The drawing under review shows one solid part. Ordinate dimensions are in mm from its lowest x, y, z. A direction names the side the tool comes from. Round coordinates to 2 decimals unless told otherwise and drop trailing zeros. Write each loop counter-clockwise with the first axis right and the second up, starting at its lowest first coordinate (ties: lowest second). Pieces come first, ordered by that corner, then holes. Notation, with made-up numbers: M 42.5,-24.5 L 79.5,-24.5 A28 cw 79.5,-4.5 Z; hole C 8,87 d10. An arc over 180 degrees is marked long. Write item = value, one per line. Start each with the question number.
Item 1: To check wall thickness, follow line 1 along Z through (x, y) = (5, 4); line 2 along Y through (x, z) = (3.5, 6); line 3 along X through (y, z) = (6, 6.25). State the ranges of each line that lie inside material, in increasing order.
Item 2: Take a section at D-D, the plane x = 1.5. Give the boundary of the cut face in (y, z), plus the area to 3 significant figures.
Item 3: Tool access review of the marked faces 1 and 2: name each direction out of +Z, -Z, +X, -X, +Y, -Y from which nothing blocks a thin tool from reaching the whole face with its end or side.
Item 4: For pin 1 Ø2 at (y, z) = (1, 1.5) entering from -X; pin 2 Ø4 at (x, y) = (4, 7) entering from +Z; pin 3 Ø1.5 at (x, y) = (4.5, 7) entering from -Z, all flat-tipped, find the tip position at first contact; note any pin that passes through.
Item 5: Take a section at C-C, the plane z = 5. Give the boundary of the cut face in (x, y).
Item 6: Take a section at B-B, the plane y = 7.75. Give the boundary of the cut face in (x, z), plus the area to 3 significant figures.
Item 7: Take a section at A-A, the plane x = 5. Give the boundary of the cut face in (y, z), plus the area to 3 significant figures.
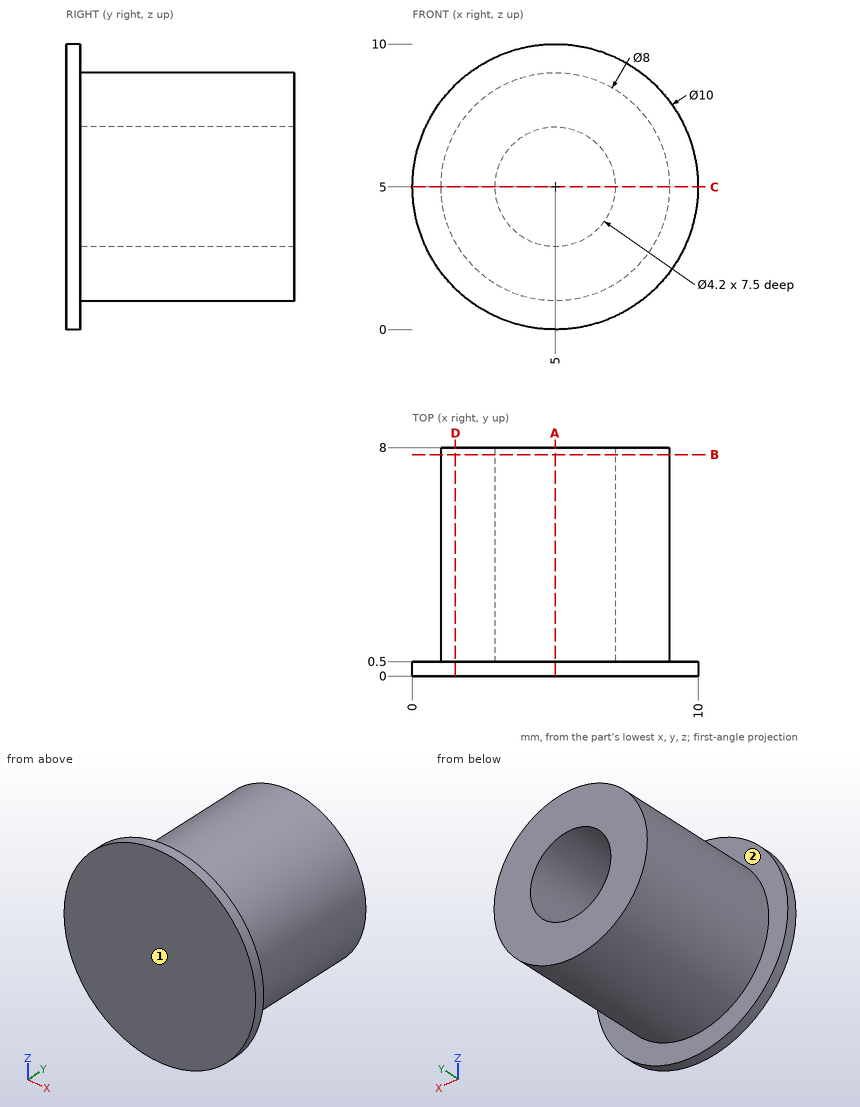
Response values:
q1.line_1 = 1 to 2.9, 7.1 to 9
q1.line_2 = 0 to 0.5
q1.line_3 = 1.2 to 3.31, 6.69 to 8.8
q2.outline = M 0,1.43 L 0.5,1.43 L 0.5,3.06 L 8,3.06 L 8,6.94 L 0.5,6.94 L 0.5,8.57 L 0,8.57 Z
q2.area = 32.6 mm2
q3.face_1 = +Z, -Z, +X, -X, -Y
q3.face_2 = +Y
q4.pin_1 = 0.75
q4.pin_2 = 9
q4.pin_3 = 1
q5.outline = M 0,0 L 10,0 L 10,0.5 L 9,0.5 L 9,8 L 7.1,8 L 7.1,0.5 L 2.9,0.5 L 2.9,8 L 1,8 L 1,0.5 L 0,0.5 Z
q6.outline = C 5,5 d8; hole C 5,5 d4.2
q6.area = 36.4 mm2
q7.outline = M 0,0 L 0.5,0 L 0.5,1 L 8,1 L 8,2.9 L 0.5,2.9 L 0.5,7.1 L 8,7.1 L 8,9 L 0.5,9 L 0.5,10 L 0,10 Z
q7.area = 33.5 mm2
